Could you check a few things on this drawing? It's one solid part, dimensions in mm from its lowest x, y, z. Round coordinates to 2 decimals unless told otherwise and drop trailing zeros. Write each loop counter-clockwise with the first axis right and the second up, starting at its lowest first coordinate (ties: lowest second). Pieces come first, ordered by that corner, then holes. Notation, with made-up numbers: (55, 12.25) - (82, 12.25) arc R30 cw to (82, 35.25) - close; hole circle Ø7 at (-6.75, -39). An arc over 180 degrees is marked (long way). Use one line per item in the form item = value. Start each with the question number.
1. Will these pins go through, and if not, where does the flat tip stop? pin 1 (4 mm diameter, centred on x = 188.91, y = 76.64, fed in from +Z); pin 2 (4 mm diameter, centred on x = 82.5, z = 33.5, fed in from -Y); pin 3 (3 mm diameter, centred on x = 71, y = 30, fed in from +Z); pin 4 (4 mm diameter, centred on x = 102, y = 44, fed in from +Z) (1 decimal).
2. I want a section at B-B, the plane z = 93.5. List the corners of the cut face in (x, y) for me.
3. I want a section at D-D, the plane x = 86.5. List the corners of the cut face in (y, z) for me, plus the area to 3 significant figures.
4. We'd pull the mould along X, two halves only. Please class the marked faces 1, 2 and 3: +X half, -X half, draft (parallel to the pull), parting line (faces both ways), or undercut.
5. If I drill on line 1 along Z through (x, y) = (99, 38) (1 decimal); line 2 along Z through (x, y) = (90.5, 19); line 3 along X through (y, z) = (71.5, 128.5), over which ranges is the centre line in solid material (lowest first)?
6. I want a section at C-C, the plane x = 147. List the corners of the cut face in (y, z) for me, plus the area to 3 significant figures.
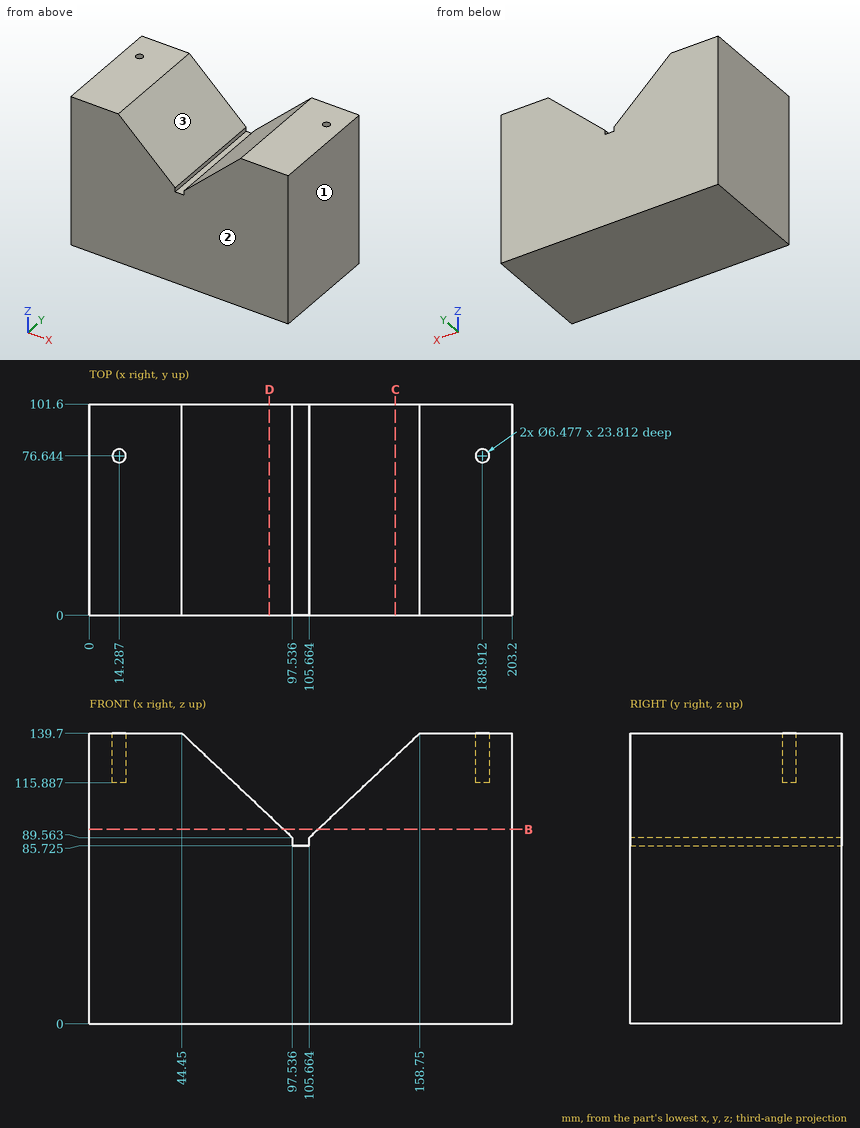
Model answer:
q1.pin_1 = 115.89
q1.pin_2 = 0
q1.pin_3 = 116.04
q1.pin_4 = 85.7
q2.outline = (0, 0) - (93.37, 0) - (93.37, 101.6) - (0, 101.6) - close; (109.83, 0) - (203.2, 0) - (203.2, 101.6) - (109.83, 101.6) - close
q3.outline = (0, 0) - (101.6, 0) - (101.6, 99.99) - (0, 99.99) - close
q3.area = 10,200 mm2
q4.face_1 = +X half
q4.face_2 = draft
q4.face_3 = undercut
q5.line_1 = 0 to 85.7
q5.line_2 = 0 to 96.21
q5.line_3 = 0 to 56.31, 146.89 to 203.2
q6.outline = (0, 0) - (101.6, 0) - (101.6, 128.6) - (0, 128.6) - close
q6.area = 13,100 mm2
